Could you check a few things on this model? Use its own coordinates, in mm. A direction names the side the tool comes from. Give positions to 0.01 mm unless a question says otherwise; leave off trailing zeros. Loops run counter-clockwise (first coordinate to the right, second up) from the corner with the lowest first, then second, coordinate; pieces in that order, holes last. Notation, with made-up numbers: M -20,60 L -12,60 A6 cw -12,69 Z; hole C 17,56.25 d7. An arc over 180 degrees is marked long. Return JSON: item names as keys, results as strings. Group by question number.
1. If we section it at C-C (y = -7.25): Write out the boundary of the cut face in (x, z), plus the area to 3 significant figures.
2. If we mould it in two halves opening along X, with no side actions, what happens to faces 1 (the flat face through (15, -15, 0)), 2 (the flat face through (-4, 0, 4)), 3 (the cylindrical face through (-1.08, -15.21, -4.88))? For each: +X half, -X half, draft (parallel to the pull), parting line (faces both ways), or undercut.
3. If we section it at A-A (x = 0): Write out the boundary of the cut face in (y, z), plus the area to 3 significant figures.
4. Please list where these lines run through material, in increasing order: line 1 (Z direction, x = 0, y = -22.5); line 2 (Z direction, x = 0, y = -14.5); line 3 (X direction, y = -13.75, z = 37).
5. For faces 4 (the flat face through (0, -15, -15)), 5 (the flat face through (-4, -18, 15)), which set-ups out of +Z, -Z, +X, -X, +Y, -Y let a thin tool reach every point of the face, with its end or its side?
6. For pin 1 (1 mm diameter, centred on x = 3.5, y = -20, fed in from +Z); pin 2 (12 mm diameter, centred on x = 11, z = -7.5, fed in from +Y), each with a flat end and sliding along its axis, tell me the tip position at first contact or that it passes through.
7. If we section it at D-D (x = -9): Write out the boundary of the cut face in (y, z).
8. If we section it at B-B (z = 0): Write out the boundary of the cut face in (x, y), plus the area to 3 significant figures.
```python
from build123d import *

# Parameters (mm, degrees)
F0_W     = 30
F0_H     = 30
F1_DEPTH = 30
F3_R     = 5
F4_DEPTH = 30.2
F5_R     = 5
F6_DEPTH = 30


with BuildPart() as f1:
    # F0 (on Front) → F1 (new body)
    with BuildSketch(Plane.XZ):
        Rectangle(F0_W, F0_H)
    extrude(amount=F1_DEPTH)

    # F3 (on face) → F4 (cut)
    with BuildSketch(Plane.XZ.offset(30)):
        Circle(F3_R)
    extrude(amount=-F4_DEPTH, mode=Mode.SUBTRACT)

    # F5 (on face) → F6 (join)
    with BuildSketch(Plane.XY.offset(15)):
        with Locations((0, -13.743456)):
            Circle(F5_R)
    extrude(amount=F6_DEPTH)


solid = f1.part
```
Answer:
{
 "1": {"outline": "M -15,-15 L 15,-15 L 15,15 L -15,15 Z; hole C 0,0 d10", "area": "821 mm²"},
 "2": {"face 1": "+X half", "face 2": "draft", "face 3": "undercut"},
 "3": {"outline": "M -30,-15 L 0,-15 L 0,-5 L -30,-5 Z; M -30,5 L 0,5 L 0,15 L -8.74,15 L -8.74,45 L -18.74,45 L -18.74,15 L -30,15 Z", "area": "900 mm²"},
 "4": {"line 1": "z = -15 to -5, 5 to 15", "line 2": "z = -15 to -5, 5 to 45", "line 3": "x = -5 to 5"},
 "5": {"face 4": "-Z, +X, -X, +Y, -Y", "face 5": "+Z"},
 "6": {"pin 1": "stops at z = 15", "pin 2": "stops at y = 0"},
 "7": {"outline": "M -30,-15 L 0,-15 L 0,15 L -30,15 Z"},
 "8": {"outline": "M -15,-30 L -5,-30 L -5,0 L -15,0 Z; M 5,-30 L 15,-30 L 15,0 L 5,0 Z", "area": "600 mm²"}
}
